Verification items for the finished model (mm, model axes). Coordinates: 2 decimals unless noted, no trailing zeros. Loops run counter-clockwise (first coordinate to the right, second up) from the corner with the lowest first, then second, coordinate; pieces in that order, holes last.
Q1. Material ranges on probe 1 along X at (y, z) = (1.75, 9); probe 2 along X at (y, z) = (2.5, -9); probe 3 along Z at (x, y) = (-98, 6), recorded low to high.
Q2. Sectioned sample at B-B (z = -111.5). Enter the section's corners in (x, y).
Q3. Sectioned sample at A-A (y = 4.75). Enter the section's corners in (x, z).
Q4. Sectioned sample at C-C (x = 97). Enter the section's corners in (y, z), then the cut area to 3 significant figures.
Q5. Go/stop test with flat-tipped pins: P1, Ø3.5, axis at x = -102.46, z = 59.16, coming from the +Y side; P2, Ø3, axis at x = -17, y = 3.5, coming from the -Z side; P3, Ø3, axis at y = 2.5, z = 4.5, coming from the -X side; P4, Ø3, axis at y = 2.5, z = 28, coming from the +X side. Record where each tip stops, or that it passes through.
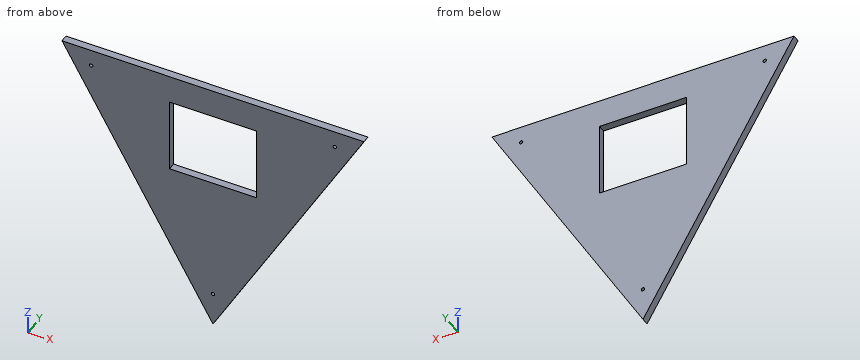
```python
from build123d import *

# Parameters (mm, degrees)
BOSS_EXTRUDE1_DEPTH = 6.35
SKETCH2_W           = 36.5
SKETCH2_H           = 63
SKETCH2_R           = 1.4224
CUT_EXTRUDE2_DEPTH  = 195.099602868


with BuildPart() as part:
    # Sketch1 → Boss-Extrude1 (new body)
    with BuildSketch(Plane(origin=(0, 0, 0), x_dir=(1, 0, 0), z_dir=(0, 1, 0))):
        Polygon((0, 146.646968374), (-127, -73.323484187), (127, -73.323484187), align=None)
    extrude(amount=BOSS_EXTRUDE1_DEPTH)

    # Sketch2 → Cut-Extrude2 (cut, through all)
    with BuildSketch(Plane(origin=(0, 6.35, 0), x_dir=(1, 0, 0), z_dir=(0, 1, 0))):
        with Locations((-18.25, -17.853484187)):
            Rectangle(SKETCH2_W, SKETCH2_H)
        with Locations((18.25, -17.853484187)):
            Rectangle(SKETCH2_W, SKETCH2_H)
        with Locations(Location((0, 118.312139176, 0), (0, 0, 270))):
            Circle(SKETCH2_R)
        with Locations(Location((-102.461318102, -59.156069588, 0), (0, 0, 270))):
            Circle(SKETCH2_R)
        with Locations(Location((102.461318102, -59.156069588, 0), (0, 0, 270))):
            Circle(SKETCH2_R)
    extrude(amount=-CUT_EXTRUDE2_DEPTH, mode=Mode.SUBTRACT)


solid = part.part
```
Geometry check:
1. probe 1: x = -89.86 to -36.5, 36.5 to 89.86
1. probe 2: x = -79.47 to -36.5, 36.5 to 79.47
1. probe 3: z = 23.09 to 73.32
2. outline: (-20.29, 0) - (20.29, 0) - (20.29, 6.35) - (-20.29, 6.35) - close
3. outline: (-127, 73.32) - (0, -146.65) - (127, 73.32) - close; hole circle Ø2.84 at (-102.46, 59.16); hole (-36.5, -13.65) - (36.5, -13.65) - (36.5, 49.35) - (-36.5, 49.35) - close; hole circle Ø2.84 at (0, -118.31); hole circle Ø2.84 at (102.46, 59.16)
4. outline: (0, 21.36) - (6.35, 21.36) - (6.35, 73.32) - (0, 73.32) - close
4. area: 330 mm2
5. P1: stops at y = 6.35
5. P2: stops at z = -119.8
5. P3: stops at x = -88.13
5. P4: stops at x = 101.7
